Build history of the part. All positions in model axes, mm. Face numbers are marked on the shaded views. A direction names the side the tool comes from. Round coordinates to 2 decimals unless told otherwise and drop trailing zeros. Loops run counter-clockwise (first coordinate to the right, second up) from the corner with the lowest first, then second, coordinate; pieces in that order, holes last. Notation, with made-up numbers: (80, 11) -> (132, 11) arc R22 cw to (132, 21) -> close; hole circle Ø8 at (13, -22). An arc over 180 degrees is marked (long way). Put each result on its own line as item: value. Start each with the question number.
Item 1: Cut at B-B, the plane y = 10.5. List the corners of the cut face in (x, z).
Item 2: Cut at D-D, the plane z = 1. Count the separate pieces of the cut face and the enclosed holes in it, plus the area to 3 significant figures.
Item 3: Pull direction X, two halves, no side cores. Call the marked faces 3 and 4: +X half, -X half, draft (parallel to the pull), parting line (faces both ways), or undercut.
Item 4: Tool access for the marked faces 1 and 2: list every direction of +Z, -Z, +X, -X, +Y, -Y with a clear straight run to the whole face (end or side of a thin tool).
Item 5: Cut at A-A, the plane x = 0. List the corners of the cut face in (y, z), plus the area to 3 significant figures.
Item 6: Flat gauge pins, fed straight in: pin 1 Ø2 at (x, z) = (34, 17) entering from -Y; pin 2 Ø5 at (y, z) = (21.5, 6) entering from -X; pin 3 Ø10 at (y, z) = (6.5, 11) entering from -X. Where does each tip first touch, or does it go through?
Item 7: Drill centre lines: probe 1 along X at (y, z) = (15, 0); probe 2 along Z at (x, y) = (0, 20.25); probe 3 along X at (y, z) = (-0.4, 0). Where is each one in solid material? Low to high. Write a range as [from, to].
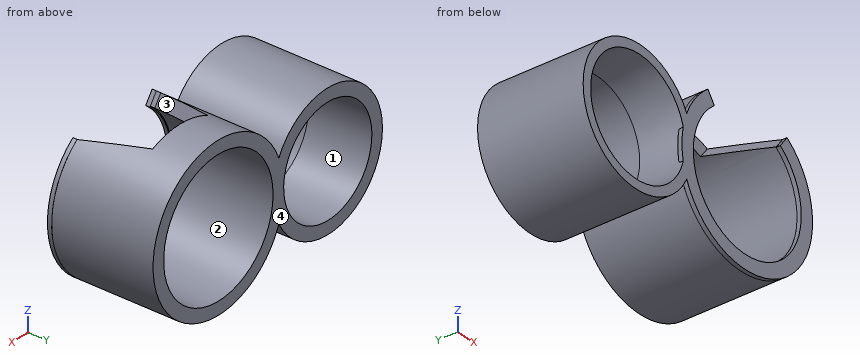
```python
from build123d import *

# Parameters (mm, degrees)
BOSS_EXTRU_6_DEPTH      = 24
BOSS_EXTRU_6_DEPTH_BACK = 1
ESQUISSE2_R             = 15.5
ESQUISSE2_R_2           = 12.5
ESQUISSE3_R             = 18.5
ESQUISSE3_R_2           = 15.5
BOSS_EXTRU_7_DEPTH      = 24
ENL_V_MAT_EXTRU_4_DEPTH = 15
CHANFREIN4_SIZE         = 4
CHANFREIN4_SIZE2        = 13.949657775
CHANFREIN5_SIZE         = 4
CHANFREIN5_SIZE2        = 14.92820323
BOSS_EXTRU_9_DEPTH      = 1


with BuildPart() as part:
    # Esquisse2 → Boss.-Extru.6 (new, two sides: drawn at the far end of the back side and taken through both)
    with BuildSketch(Plane(origin=(0, 0, 0), x_dir=(1, 0, 0), z_dir=(0, 1, 0)).offset(-BOSS_EXTRU_6_DEPTH_BACK)):
        with Locations(Location((0, 0, 0), (0, 0, 270))):
            Circle(ESQUISSE2_R)
        with Locations(Location((0, 0, 0), (0, 0, 270))):
            Circle(ESQUISSE2_R_2, mode=Mode.SUBTRACT)
    extrude(amount=BOSS_EXTRU_6_DEPTH + BOSS_EXTRU_6_DEPTH_BACK)

    # Esquisse3 → Boss.-Extru.7 (add)
    with BuildSketch(Plane(origin=(0, 0, 0), x_dir=(1, 0, 0), z_dir=(0, 1, 0))):
        with Locations((31, 0)):
            Circle(ESQUISSE3_R)
        with Locations(Location((31, 0, 0), (0, 0, 179.99985447))):
            Circle(ESQUISSE3_R_2, mode=Mode.SUBTRACT)
    extrude(amount=BOSS_EXTRU_7_DEPTH)

    # Esquisse6 → Enl_v. mat.-Extru.4 (cut)
    with BuildSketch(Plane(origin=(0, 0, 0), x_dir=(1, 0, 0), z_dir=(0, 1, 0))):
        with BuildLine():
            Line((21.542410955, -12.280228396), (19.846119293, -14.759435801))
            ThreePointArc((19.846119293, -14.759435801), (31.084403323, -18.499807461), (42.288090151, -14.657046795))
            Line((42.288090151, -14.657046795), (40.457589045, -12.280228396))
            ThreePointArc((40.457589045, -12.280228396), (31, -15.5), (21.542410955, -12.280228396))
        make_face()
    extrude(amount=ENL_V_MAT_EXTRU_4_DEPTH, mode=Mode.SUBTRACT)

    # Chanfrein3: read off the stored shape, not the designer's step
    # Chanfrein3 outline → Chanfrein3 (revolve, cut)
    with BuildSketch(Plane.XY):
        Polygon((13.374886635, -1), (12.5, 9), (12.5, -1), align=None)
    revolve(axis=Axis((0, 0, 0), (0, 1, 0)), mode=Mode.SUBTRACT)

    # Chanfrein4
    chanfrein4_edges = [part.edges().sort_by_distance(p)[0] for p in [
        (20.694265124, 15, 13.519832098),
    ]]
    chanfrein4_side = [part.faces().sort_by_distance(p)[0] for p in [
        (31.040377675, 15, 15.854130796),
    ]]
    chamfer(chanfrein4_edges, length=CHANFREIN4_SIZE, length2=CHANFREIN4_SIZE2, reference=chanfrein4_side[0])

    # Chanfrein5
    chanfrein5_edges = [part.edges().sort_by_distance(p)[0] for p in [
        (41.372839598, 15, 13.468637595),
    ]]
    chanfrein5_side = [part.faces().sort_by_distance(p)[0] for p in [
        (32.951306309, 15, 16.129493261),
    ]]
    chamfer(chanfrein5_edges, length=CHANFREIN5_SIZE, length2=CHANFREIN5_SIZE2, reference=chanfrein5_side[0])

    # Esquisse18 → Boss.-Extru.9 (add)
    with BuildSketch(Plane(origin=(0, 0, 0), x_dir=(1, 0, 0), z_dir=(0, 1, 0))):
        with BuildLine():
            Line((40.360227094, -12.108845331), (42.293943816, -14.6646475))
            ThreePointArc((42.293943816, -14.6646475), (30.929770772, 18.504604183), (19.846119293, -14.759435801))
            Line((19.846119293, -14.759435801), (21.667455033, -12.118000277))
            ThreePointArc((21.667455033, -12.118000277), (31.000415105, 15.299998165), (40.360227094, -12.108845331))
        make_face()
    extrude(amount=-BOSS_EXTRU_9_DEPTH)


solid = part.part
```
Reply:
1. outline: (13.85, -6.95) arc R18.5 ccw (long way) to (39.94, 16.19) -> (38.09, 13.78) arc R15.5 cw (long way) to (23.83, 13.74) -> (22.12, 16.23) arc R18.5 ccw to (13.85, 6.95) arc R15.5 ccw (long way) to start; hole circle Ø25 at (0, 0)
2. separate pieces: 3
2. enclosed holes: 0
2. area: 220 mm^2
3. face 3: undercut
3. face 4: draft
4. face 1: +Y, -Y
4. face 2: +Y
5. outline: (-1, -15.5) -> (24, -15.5) -> (24, -12.5) -> (9, -12.5) -> (-1, -13.37) -> close; (-1, 13.37) -> (9, 12.5) -> (24, 12.5) -> (24, 15.5) -> (-1, 15.5) -> close
5. area: 141 mm^2
6. pin 1: stops at y = 15
6. pin 2: stops at x = -15.1
6. pin 3: stops at x = -14.29
7. probe 1: x = [-15.5, -12.5], [12.5, 15.5], [46.5, 49.5]
7. probe 2: z = [-15.5, -12.5], [12.5, 15.5]
7. probe 3: x = [-15.5, -13.32], [12.5, 15.71], [46.31, 49.51]
